Design review of the part built by this model. Coordinates are the model's own, in mm. A direction names the side the tool comes from. Round coordinates to 2 decimals unless told otherwise and drop trailing zeros. Loops run counter-clockwise (first coordinate to the right, second up) from the corner with the lowest first, then second, coordinate; pieces in that order, holes last. Notation, with made-up numbers: (61, 24.25) -> (91, 24.25) arc R31 ccw to (91, 59.25) -> close; hole circle Ø7 at (-25, -12). An arc over 180 degrees is marked (long way). Write each question's results on one line, items separated by ' | '. Start each with the question number.
from build123d import *

# Parameters (mm, degrees)
SKETCH_1_R      = 2
EXTRUDE_1_DEPTH = 2.4
EXTRUDE_2_DEPTH = 7.3


with BuildPart() as part:
    # 草图1 → 凸台-拉伸1 (new body)
    with BuildSketch(Plane.XY):
        Circle(SKETCH_1_R)
    extrude(amount=-EXTRUDE_1_DEPTH)

    # 草图2 → 凸台-拉伸2 (add)
    with BuildSketch(Plane(origin=(0, 0, -2.4), x_dir=(-1, 0, 0), z_dir=(0, 0, -1))):
        with BuildLine():
            ThreePointArc((2, 0), (1.974474181, 0.318514847), (1.898548292, 0.628899341))
            Line((1.898548292, 0.628899341), (-1.493916952, 1.329741381))
            ThreePointArc((-1.493916952, 1.329741381), (-0.711395142, -1.869202223), (2, 0))
        make_face()
    extrude(amount=EXTRUDE_2_DEPTH)


solid = part.part
1) For faces 1 (the face through (0, 0, 0)), 2 (the face through (-0.2, 1.3, -2.4)), list the 3-axis set-ups (+Z, -Z, +X, -X, +Y, -Y) from which the entire face can be reached by the end or side of a thin tool; tool diameter is ignored.
2) Take a section at A-A (x = -0.7). Write out the cut boundary in (y, z), plus the area to 3 significant figures.
3) To check wall thickness, follow line 1 (Y direction, x = 1.65, z = -2); line 2 (X direction, y = 0.3, z = -5.5); line 3 (Y direction, x = -1, z = -4.25). State the ranges of each line that lie inside material, in increasing order. Write a range as from..to.
4) Take a section at D-D (z = -0.75). Write out the cut boundary in (x, y).
5) Take a section at C-C (x = 0.15). Write out the cut boundary in (y, z).
6) Take a section at B-B (z = -7). Write out the cut boundary in (x, y).
Geometry check:
1) face 1: +Z, +X, -X, +Y, -Y | face 2: -Z, -X, +Y
2) outline: (-1.87, -9.7) -> (0.88, -9.7) -> (0.88, -2.4) -> (1.87, -2.4) -> (1.87, 0) -> (-1.87, 0) -> close | area: 29.1 mm^2
3) line 1: y = -1.13..1.13 | line 2: x = -1.98..1.98 | line 3: y = -1.73..0.81
4) outline: circle Ø4 at (0, 0)
5) outline: (-1.99, -9.7) -> (1.05, -9.7) -> (1.05, -2.4) -> (1.99, -2.4) -> (1.99, 0) -> (-1.99, 0) -> close
6) outline: (-1.9, 0.63) arc R2 ccw (long way) to (1.49, 1.33) -> close
